For this review, take the finished solid that the model builds, in its own axes (mm). Give positions to 0.01 mm unless a question says otherwise; leave off trailing zeros. Loops run counter-clockwise (first coordinate to the right, second up) from the corner with the lowest first, then second, coordinate; pieces in that order, holes last.
```python
from build123d import *

# Parameters (mm, degrees)
SKETCH_1_R          = 1
EXTRUDE_1_DEPTH     = 2
FILLET_1_R          = 3
CUT_EXTRUDE_1_DEPTH = 10
OTHER_1_DEPTH       = 2


# Read off the part's stored shape, not the designer's step: 填充阵列1
with BuildPart() as part:
    # 草图1 → 凸台-拉伸1 (new body)
    with BuildSketch(Plane.XY):
        Polygon((-246.460434143, 16.421045692), (-247.367512812, -43.383226063), (-279.241752663, -42.899690556), (-278.334515728, 16.904578798), align=None)
        with Locations((-273.852745372, 10.835899523)):
            Circle(SKETCH_1_R, mode=Mode.SUBTRACT)
        with Locations((-253.855045493, 10.532585287)):
            Circle(SKETCH_1_R, mode=Mode.SUBTRACT)
        with Locations((-254.580263739, -37.273170465)):
            Circle(SKETCH_1_R, mode=Mode.SUBTRACT)
        with Locations((-274.577962013, -36.969750385)):
            Circle(SKETCH_1_R, mode=Mode.SUBTRACT)
    extrude(amount=EXTRUDE_1_DEPTH)

    # 圆角1
    fillet_1_edges = [part.edges().sort_by_distance(p)[0] for p in [
        (-246.460434143, 16.421045692, 1),
        (-247.367512812, -43.383226063, 1),
        (-279.241752663, -42.899690556, 1),
        (-278.334515728, 16.904578798, 1),
    ]]
    fillet(fillet_1_edges, radius=FILLET_1_R)

    # 草图2 → 切除-拉伸1 (cut)
    with BuildSketch(Plane.XY.offset(2)):
        Polygon((-260.851053776, -13.269658771), (-264.851053776, -13.208979355), (-264.851053776, -14.394019601), (-262.851053776, -15.54872014), (-260.851053776, -14.394019601), align=None)
        Polygon((-264.851053776, -12.084618525), (-264.851053776, -13.208979355), (-260.851053776, -13.269658771), (-260.851053776, -12.084618525), (-262.851053776, -10.929917986), align=None)
    extrude(amount=-CUT_EXTRUDE_1_DEPTH, mode=Mode.SUBTRACT)

    # 填充阵列1 outline → 填充阵列1 (cut)
    with BuildSketch(Plane.XY):
        Polygon((-258.52417318, 5.321431628), (-258.52417318, 3.012030551), (-256.52417318, 1.857330013), (-254.52417318, 3.012030551), (-254.52417318, 5.321431628), (-256.52417318, 6.476132167), align=None)
        Polygon((-271.07177439, -22.49147372), (-271.07177439, -24.800874796), (-269.07177439, -25.955575335), (-267.07177439, -24.800874796), (-267.07177439, -22.49147372), (-269.07177439, -21.336773181), align=None)
        Polygon((-258.94881311, -22.675348203), (-258.94881311, -24.98474928), (-256.94881311, -26.139449818), (-254.94881311, -24.98474928), (-254.94881311, -22.675348203), (-256.94881311, -21.520647665), align=None)
        Polygon((-264.957213759, -19.083813483), (-264.957213759, -21.393214559), (-262.957213759, -22.547915098), (-260.957213759, -21.393214559), (-260.957213759, -19.083813483), (-262.957213759, -17.929112944), align=None)
        Polygon((-270.965614407, -15.492278762), (-270.965614407, -17.801679839), (-268.965614407, -18.956380377), (-266.965614407, -17.801679839), (-266.965614407, -15.492278762), (-268.965614407, -14.337578223), align=None)
        Polygon((-265.063373741, -26.08300844), (-265.063373741, -28.392409517), (-263.063373741, -29.547110056), (-261.063373741, -28.392409517), (-261.063373741, -26.08300844), (-263.063373741, -24.928307902), align=None)
        Polygon((-259.054973093, -29.674543161), (-259.054973093, -31.983944238), (-257.054973093, -33.138644776), (-255.054973093, -31.983944238), (-255.054973093, -29.674543161), (-257.054973093, -28.519842623), align=None)
        Polygon((-271.177934372, -29.490668678), (-271.177934372, -31.800069754), (-269.177934372, -32.954770293), (-267.177934372, -31.800069754), (-267.177934372, -29.490668678), (-269.177934372, -28.335968139), align=None)
        Polygon((-270.753294442, -1.493888846), (-270.753294442, -3.803289923), (-268.753294442, -4.957990461), (-266.753294442, -3.803289923), (-266.753294442, -1.493888846), (-268.753294442, -0.339188308), align=None)
        Polygon((-258.630333163, -1.67776333), (-258.630333163, -3.987164406), (-256.630333163, -5.141864945), (-254.630333163, -3.987164406), (-254.630333163, -1.67776333), (-256.630333163, -0.523062791), align=None)
        Polygon((-264.638733811, 1.913771391), (-264.638733811, -0.395629686), (-262.638733811, -1.550330224), (-260.638733811, -0.395629686), (-260.638733811, 1.913771391), (-262.638733811, 3.068471929), align=None)
        Polygon((-270.647134459, 5.505306112), (-270.647134459, 3.195905035), (-268.647134459, 2.041204497), (-266.647134459, 3.195905035), (-266.647134459, 5.505306112), (-268.647134459, 6.66000665), align=None)
        Polygon((-258.842653128, -15.676153245), (-258.842653128, -17.985554322), (-256.842653128, -19.14025486), (-254.842653128, -17.985554322), (-254.842653128, -15.676153245), (-256.842653128, -14.521452707), align=None)
        Polygon((-270.859454424, -8.493083804), (-270.859454424, -10.802484881), (-268.859454424, -11.957185419), (-266.859454424, -10.802484881), (-266.859454424, -8.493083804), (-268.859454424, -7.338383266), align=None)
        Polygon((-258.736493145, -8.676958287), (-258.736493145, -10.986359364), (-256.736493145, -12.141059903), (-254.736493145, -10.986359364), (-254.736493145, -8.676958287), (-256.736493145, -7.522257749), align=None)
        Polygon((-264.744893794, -5.085423567), (-264.744893794, -7.394824644), (-262.744893794, -8.549525182), (-260.744893794, -7.394824644), (-260.744893794, -5.085423567), (-262.744893794, -3.930723028), align=None)
    extrude(amount=OTHER_1_DEPTH, mode=Mode.SUBTRACT)


solid = part.part
```
Item 1: Take a section at A-A on y = -3. Give the boundary of the cut face in (x, z) (3 decimals).
Answer:
outline: (-278.636, 0) - (-270.753, 0) - (-270.753, 2) - (-278.636, 2) - close; (-266.753, 0) - (-258.63, 0) - (-258.63, 2) - (-266.753, 2) - close; (-254.63, 0) - (-246.755, 0) - (-246.755, 2) - (-254.63, 2) - close
Item 2: The part is to be moulded in two halves that separate along Y. For faces 1 (the flat face through (-259, -13, 2)), 2 (the flat face through (-269.77, -4.37, 0.99)), 3 (the cylindrical face through (-277.445, 16.036, 1.014)), 4 (the flat face through (-255.64, -4.57, 0.99)), say which applies: released by +Y, released by -Y, zero draft, split by the parting line, or undercut.
Answer:
face 1: zero draft
face 2: undercut
face 3: released by +Y
face 4: undercut
Item 3: For L1, parallel to X at y = 5, z = 0.15; L2, parallel to Y at x = -254, z = 0.4; L3, parallel to X at y = -2, z = 1.05, list the stretches that pass through material, from the lowest coordinate up.
Answer:
L1: x = -278.52 to -270.65, -266.65 to -258.52, -254.52 to -246.63
L2: y = -43.28 to -38.09, -36.46 to 9.54, 11.52 to 16.54
L3: x = -278.62 to -270.75, -266.75 to -258.63, -254.63 to -246.74
Item 4: Clearance check with flat-ended pins moving along their axes: pin 1 Ø1 at (y, z) = (4.5, 1.5) entering from +X; pin 2 Ø0.6 at (y, z) = (-20.5, 1) entering from +X; pin 3 Ø1.8 at (x, y) = (-253.86, 10.53) entering from -Z; pin 4 Ø1 at (x, z) = (-272.5, 1) entering from -Y. State where each tip first meets the part, or that it passes through.
Answer:
pin 1: stops at x = -246.63
pin 2: stops at x = -247.02
pin 3: passes through
pin 4: stops at y = -43.01
Item 5: Take a section at B-B on z = 1.35. State how many separate pieces and enclosed holes the cut face has, and give its area (3 significant figures).
Answer:
separate pieces: 1
enclosed holes: 21
area: 1,650 mm2
